from build123d import *

# Parameters (mm, degrees)
SKETCH1_R           = 1.5
SKETCH1_R_2         = 1.9
SKETCH1_W           = 12
SKETCH1_H           = 8.4
BOSS_EXTRUDE1_DEPTH = 3


with BuildPart() as part:
    # Sketch1 → Boss-Extrude1 (new body)
    with BuildSketch(Plane(origin=(0, 0, 0), x_dir=(1, 0, 0), z_dir=(0, 1, 0))):
        with BuildLine():
            Line((-19.05, 10), (19.05, 10))
            ThreePointArc((19.05, 10), (29.05, 0), (19.05, -10))
            Line((19.05, -10), (-19.05, -10))
            ThreePointArc((-19.05, -10), (-29.05, 0), (-19.05, 10))
        make_face()
        with Locations(Location((-9.73765424, 0, 0), (0, 0, 270))):
            Circle(SKETCH1_R, mode=Mode.SUBTRACT)
        with Locations(Location((-19.05, 0, 0), (0, 0, 270))):
            Circle(SKETCH1_R_2, mode=Mode.SUBTRACT)
        with Locations(Location((19.05, 0, 0), (0, 0, 270))):
            Circle(SKETCH1_R_2, mode=Mode.SUBTRACT)
        with Locations((4.854803124, 0)):
            Rectangle(SKETCH1_W, SKETCH1_H, mode=Mode.SUBTRACT)
    extrude(amount=BOSS_EXTRUDE1_DEPTH)


solid = part.part
Verification items for the finished model (mm, model axes). A direction names the side the tool comes from. Round coordinates to 2 decimals unless told otherwise and drop trailing zeros. Order: outer loops, then holes, each group sorted by start corner. A loop starts at its lowest first (then second) coordinate and runs counter-clockwise, first axis right, second up.
1. Section check A-A on x = 3.5. Record the cut outline in (y, z), then the cut area to 3 significant figures.
Final values:
outline: (0, -10) - (3, -10) - (3, -4.2) - (0, -4.2) - close; (0, 4.2) - (3, 4.2) - (3, 10) - (0, 10) - close
area: 34.8 mm2
2. Thickness scan on L1, parallel to X at y = 1.25, z = 0; L2, parallel to Z at x = 4.5, y = 2.3; L3, parallel to X at y = 2.4, z = 0.5. Record the ranges inside material, lowest first.
Final values:
L1: x = -29.05 to -20.95, -17.15 to -11.24, -8.24 to -1.15, 10.85 to 17.15, 20.95 to 29.05
L2: z = -10 to -4.2, 4.2 to 10
L3: x = -29.04 to -20.88, -17.22 to -11.15, -8.32 to -1.15, 10.85 to 17.22, 20.88 to 29.04
3. Section check B-B on z = 0. Record the cut outline in (x, y).
Final values:
outline: (-29.05, 0) - (-20.95, 0) - (-20.95, 3) - (-29.05, 3) - close; (-17.15, 0) - (-11.24, 0) - (-11.24, 3) - (-17.15, 3) - close; (-8.24, 0) - (-1.15, 0) - (-1.15, 3) - (-8.24, 3) - close; (10.85, 0) - (17.15, 0) - (17.15, 3) - (10.85, 3) - close; (20.95, 0) - (29.05, 0) - (29.05, 3) - (20.95, 3) - close
4. Access from +Z, -Z, +X, -X, +Y, -Y to the whole of each face (thin tool, end or side, straight path). Record for faces 4 (the cylindrical face through (-29.048, 1.479, 0.22)), 5 (the flat face through (10.855, 1, 0)).
Final values:
face 4: -X, +Y, -Y
face 5: +Y, -Y
5. Release check for a two-part mould opening along Z. For faces 1 (the cylindrical face through (20.934, 1.479, -0.247)), 2 (the flat face through (0, 0, -5)), 3 (the flat face through (0, 1, -10)) record: +Z half, -Z half, draft (parallel to the pull), parting line (faces both ways), or undercut.
Final values:
face 1: undercut
face 2: draft
face 3: -Z half
6. Go/stop test with flat-tipped pins: P1, Ø1.5, axis at y = 2, z = -1.5, coming from the +X side; P2, Ø1, axis at y = 1, z = 3.5, coming from the +X side. Record where each tip stops, or that it passes through.
Final values:
P1: stops at x = 29.02
P2: stops at x = 28.59
7. Section check C-C on y = 1.9. Record the cut outline in (x, z), then the cut area to 3 significant figures.
Final values:
outline: (-19.05, -10) - (19.05, -10) arc R10 ccw to (19.05, 10) - (-19.05, 10) arc R10 ccw to start; hole circle Ø3.8 at (-19.05, 0); hole circle Ø3 at (-9.74, 0); hole (-1.15, -4.2) - (10.85, -4.2) - (10.85, 4.2) - (-1.15, 4.2) - close; hole circle Ø3.8 at (19.05, 0)
area: 946 mm2
8. Section check D-D on z = 6. Record the cut outline in (x, y), then the cut area to 3 significant figures.
Final values:
outline: (-27.05, 0) - (27.05, 0) - (27.05, 3) - (-27.05, 3) - close
area: 162 mm2
